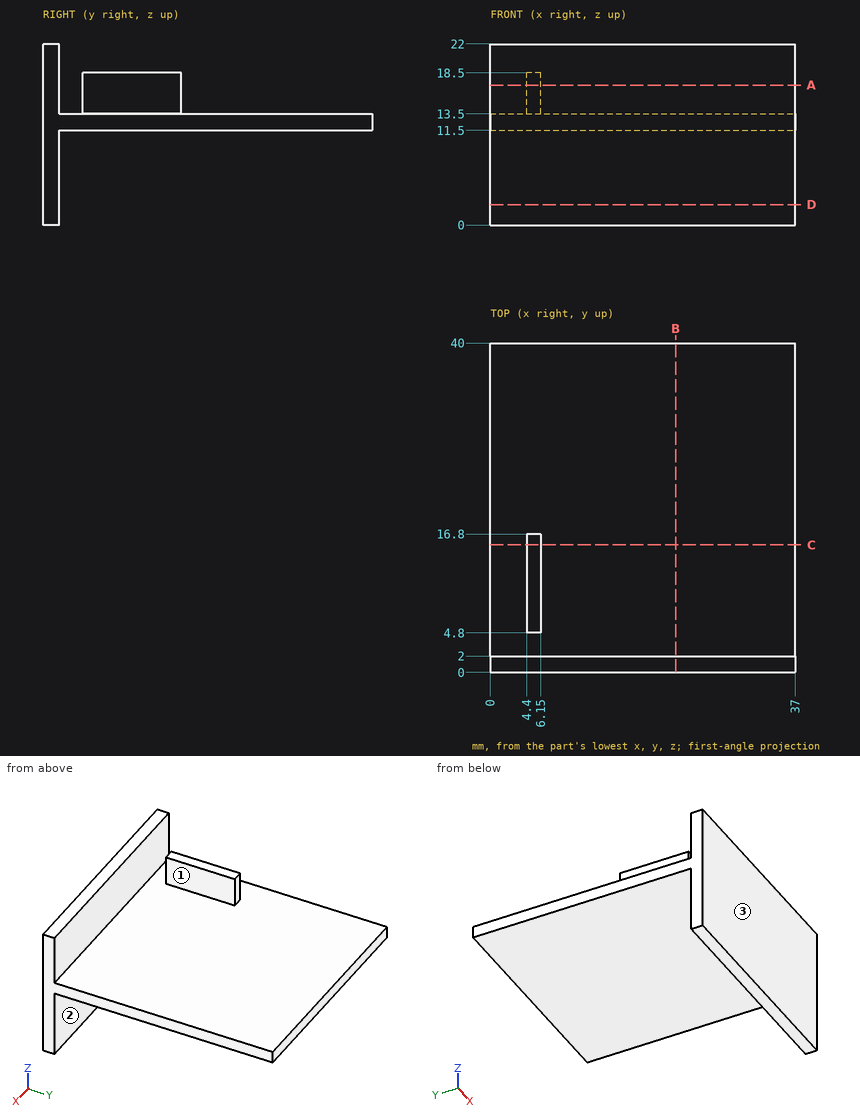
Job drawing, mm, ordinate dimensions from the low corner. One solid piece. A direction names the side the tool comes from. Round coordinates to 2 decimals unless told otherwise and drop trailing zeros. Loops run counter-clockwise (first coordinate to the right, second up) from the corner with the lowest first, then second, coordinate; pieces in that order, holes last. Notation, with made-up numbers: (40.5, 11.5) -> (50.5, 11.5) arc R20 cw to (50.5, 22.5) -> close; hole circle Ø7 at (60.25, 59.5). An arc over 180 degrees is marked (long way). One line per item, written item: value. Start each with the question number.
Q1. Cut at C-C on y = 15.5. List the corners of the cut face in (x, z), plus the area to 4 significant figures.
Q2. Cut at B-B on x = 22.5. List the corners of the cut face in (y, z), plus the area to 3 significant figures.
Q3. Probe line 1 along Y through (x, z) = (7, 6.25); line 2 along Z through (x, y) = (17.5, 24). List the from-to ranges inside material, lowest first.
Q4. Drop flat-ended pins along their axis: pin 1 Ø1 at (x, z) = (27.5, 3) entering from +Y; pin 2 Ø2.5 at (y, z) = (8, 16) entering from -X; pin 3 Ø12 at (x, y) = (30.5, 29) entering from -Z. Give the stop position or say it passes through.
Q5. 3-axis set-ups, long thin cutter, end or side, ignore diameter. For the marked faces 1, 2 and 3: which of +Z, -Z, +X, -X, +Y, -Y reach the whole face in a straight line?
Q6. Cut at A-A on z = 17. List the corners of the cut face in (x, y).
Q7. Cut at D-D on z = 2.5. List the corners of the cut face in (x, y), plus the area to 3 significant figures.
Computed:
1. outline: (0, 11.5) -> (37, 11.5) -> (37, 13.5) -> (6.15, 13.5) -> (6.15, 18.5) -> (4.4, 18.5) -> (4.4, 13.5) -> (0, 13.5) -> close
1. area: 82.75 mm²
2. outline: (0, 0) -> (2, 0) -> (2, 11.5) -> (40, 11.5) -> (40, 13.5) -> (2, 13.5) -> (2, 22) -> (0, 22) -> close
2. area: 120 mm²
3. line 1: 0 to 2
3. line 2: 11.5 to 13.5
4. pin 1: y = 2
4. pin 2: x = 4.4
4. pin 3: z = 11.5
5. face 1: +Z, +X, +Y
5. face 2: -Z, +X, -X, +Y
5. face 3: +Z, -Z, +X, -X, -Y
6. outline: (0, 0) -> (37, 0) -> (37, 2) -> (0, 2) -> close; (4.4, 4.8) -> (6.15, 4.8) -> (6.15, 16.8) -> (4.4, 16.8) -> close
7. outline: (0, 0) -> (37, 0) -> (37, 2) -> (0, 2) -> close
7. area: 74.0 mm²
